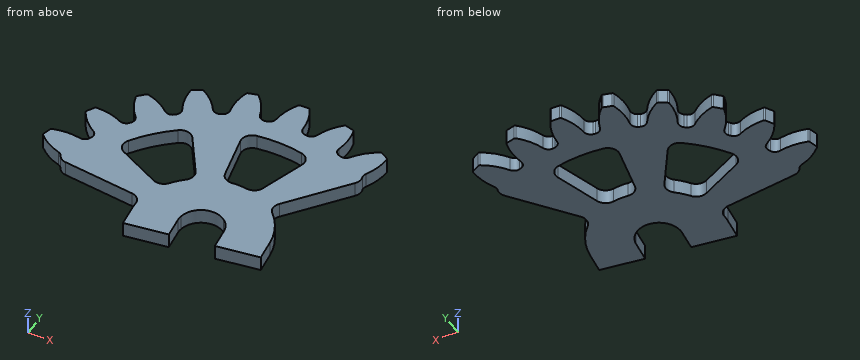
```python
from build123d import *

# Parameters (mm, degrees)
SKETCH3_R                = 136.611351841
EXTRUDE1_DEPTH           = 12.7
EXTRUDE2_DEPTH           = 12.7
FILLET2_R                = 1.5875
CIRPATTERN1_COUNT        = 24
FILLET2_OF_CIRPATTERN1_R = 1.5875
CUT_EXTRUDE1_DEPTH       = 234.890969431
CUT_EXTRUDE1_DEPTH_BACK  = 234.890969431
CUT_EXTRUDE2_REACH       = 232.646
SKETCH5_R                = 19.05
EXTRUDE3_DEPTH           = 12.7
CUT_EXTRUDE5_DEPTH       = 231.646456089
FILLET1_R                = 9.525
CUT_EXTRUDE7_DEPTH       = 12.7


with BuildPart() as part:
    # Sketch3 → Extrude1 (new body)
    with BuildSketch(Plane.XY):
        Circle(SKETCH3_R)
    extrude(amount=EXTRUDE1_DEPTH)

    # Sketch2 → Extrude2 (add)
    with BuildSketch(Plane.XY):
        with BuildLine():
            Line((-4.546074008, 165.141901983), (4.546074008, 165.141901983))
            ThreePointArc((4.546074008, 165.141901983), (9.719017906, 153.717756782), (11.846410355, 141.35876639))
            ThreePointArc((11.846410355, 141.35876639), (13.677789854, 137.226095775), (17.83135957, 135.442622788))
            Line((17.83135957, 135.442622788), (17.83135957, 110.042622788))
            Line((17.83135957, 110.042622788), (-17.83135957, 110.042622788))
            Line((-17.83135957, 110.042622788), (-17.83135957, 135.442622788))
            ThreePointArc((-17.83135957, 135.442622788), (-13.677789854, 137.226095775), (-11.846410355, 141.35876639))
            ThreePointArc((-11.846410355, 141.35876639), (-9.719017906, 153.717756782), (-4.546074008, 165.141901983))
        make_face()
    extrude2 = extrude(amount=EXTRUDE2_DEPTH)

    # Fillet2
    fillet2_edges = [part.edges().sort_by_distance(p)[0] for p in [
        (4.546074008, 165.141901983, 6.35),
        (-4.546074008, 165.141901983, 6.35),
    ]]
    fillet(fillet2_edges, radius=FILLET2_R)

    # CirPattern1: Extrude2 ×24 about axis
    cirpattern1_axis = Axis((0, 0, 0), (0, 0, 1))
    for i in range(1, CIRPATTERN1_COUNT):
        add(extrude2.rotate(cirpattern1_axis, i * 360 / CIRPATTERN1_COUNT))

    # Fillet2 of CirPattern1
    fillet2_of_cirpattern1_edges = [part.edges().sort_by_distance(p)[0] for p in [
        (-38.350699085, 160.691438662, 6.35),
        (-47.13303967, 158.338217595, 6.35),
        (-78.633935413, 145.290119351, 6.35),
        (-86.50796657, 140.744045343, 6.35),
        (-113.558398992, 119.987518509, 6.35),
        (-119.987518509, 113.558398992, 6.35),
        (-140.744045343, 86.50796657, 6.35),
        (-145.290119351, 78.633935413, 6.35),
        (-158.338217595, 47.13303967, 6.35),
        (-160.691438662, 38.350699085, 6.35),
        (-165.141901983, 4.546074008, 6.35),
        (-165.141901983, -4.546074008, 6.35),
        (-160.691438662, -38.350699085, 6.35),
        (-158.338217595, -47.13303967, 6.35),
        (-145.290119351, -78.633935413, 6.35),
        (-140.744045343, -86.50796657, 6.35),
        (-119.987518509, -113.558398992, 6.35),
        (-113.558398992, -119.987518509, 6.35),
        (-86.50796657, -140.744045343, 6.35),
        (-78.633935413, -145.290119351, 6.35),
        (-47.13303967, -158.338217595, 6.35),
        (-38.350699085, -160.691438662, 6.35),
        (-4.546074008, -165.141901983, 6.35),
        (4.546074008, -165.141901983, 6.35),
        (38.350699085, -160.691438662, 6.35),
        (47.13303967, -158.338217595, 6.35),
        (78.633935413, -145.290119351, 6.35),
        (86.50796657, -140.744045343, 6.35),
        (113.558398992, -119.987518509, 6.35),
        (119.987518509, -113.558398992, 6.35),
        (140.744045343, -86.50796657, 6.35),
        (145.290119351, -78.633935413, 6.35),
        (158.338217595, -47.13303967, 6.35),
        (160.691438662, -38.350699085, 6.35),
        (165.141901983, -4.546074008, 6.35),
        (165.141901983, 4.546074008, 6.35),
        (160.691438662, 38.350699085, 6.35),
        (158.338217595, 47.13303967, 6.35),
        (145.290119351, 78.633935413, 6.35),
        (140.744045343, 86.50796657, 6.35),
        (119.987518509, 113.558398992, 6.35),
        (113.558398992, 119.987518509, 6.35),
        (86.50796657, 140.744045343, 6.35),
        (78.633935413, 145.290119351, 6.35),
        (47.13303967, 158.338217595, 6.35),
        (38.350699085, 160.691438662, 6.35),
    ]]
    fillet(fillet2_of_cirpattern1_edges, radius=FILLET2_OF_CIRPATTERN1_R)

    # Sketch4 → Cut-Extrude1 (cut, two sides: drawn at the far end of the back side and taken through both)
    with BuildSketch(Plane.XY.offset(-CUT_EXTRUDE1_DEPTH_BACK)):
        Polygon((-1275.53694573, 167.92762467), (-268.218413087, 35.311623982), (0, 0), (164.689969961, 214.628147505), (783.198061827, 1020.683586133), (1560.818943381, -856.6592925), (-497.916064176, -1709.415253962), align=None)
    extrude(amount=CUT_EXTRUDE1_DEPTH + CUT_EXTRUDE1_DEPTH_BACK, mode=Mode.SUBTRACT)

    # Sketch5 → Cut-Extrude2 (cut, up to next)
    with BuildSketch(Plane.XY, mode=Mode.PRIVATE) as cut_extrude2_sk1:
        Circle(SKETCH5_R)
    cut_extrude2_tool1 = extrude(cut_extrude2_sk1.sketch, amount=CUT_EXTRUDE2_REACH, mode=Mode.PRIVATE) & part.part
    add(cut_extrude2_tool1.solids().sort_by_distance((0, 0, 0))[0], mode=Mode.SUBTRACT)

    # Sketch6 → Extrude3 (add)
    with BuildSketch(Plane.XY):
        with BuildLine():
            Line((-18.887024609, -2.486523962), (-16.400500647, -21.373548571))
            Line((-16.400500647, -21.373548571), (-54.174549866, -26.346596495))
            Line((-54.174549866, -26.346596495), (-56.661073828, -7.459571885))
            ThreePointArc((-56.661073828, -7.459571885), (-57.15, 0), (-56.661073828, 7.459571885))
            Line((-56.661073828, 7.459571885), (-18.887024609, 2.486523962))
            ThreePointArc((-18.887024609, 2.486523962), (-19.05, 0), (-18.887024609, -2.486523962))
        make_face()
        with BuildLine():
            Line((11.596905223, 15.113381133), (34.790715668, 45.340143398))
            ThreePointArc((34.790715668, 45.340143398), (49.493351826, 28.575), (56.661073828, 7.459571885))
            Line((56.661073828, 7.459571885), (59.147597789, -11.427452724))
            Line((59.147597789, -11.427452724), (21.373548571, -16.400500647))
            Line((21.373548571, -16.400500647), (18.887024609, 2.486523962))
            ThreePointArc((18.887024609, 2.486523962), (16.497783942, 9.525), (11.596905223, 15.113381133))
        make_face()
    extrude(amount=EXTRUDE3_DEPTH)

    # Sketch8 → Cut-Extrude5 (cut, through all)
    with BuildSketch(Plane.XY):
        with BuildLine():
            Line((-25.426243647, 114.690373436), (-12.369523937, 55.795316807))
            ThreePointArc((-12.369523937, 55.795316807), (2.492847988, 57.095605863), (17.185336442, 54.504923735))
            Line((17.185336442, 54.504923735), (35.325413797, 112.037898789))
            ThreePointArc((35.325413797, 112.037898789), (5.124187531, 117.36318983), (-25.426243647, 114.690373436))
        make_face()
        with BuildLine():
            Line((-63.119271491, 99.077410097), (-30.706672617, 48.199821128))
            ThreePointArc((-30.706672617, 48.199821128), (-42.135399799, 38.609980365), (-50.692669116, 26.388933246))
            Line((-50.692669116, 26.388933246), (-104.201597628, 54.24391834))
            ThreePointArc((-104.201597628, 54.24391834), (-86.611655142, 79.36495964), (-63.119271491, 99.077410097))
        make_face()
    extrude(amount=CUT_EXTRUDE5_DEPTH, mode=Mode.SUBTRACT)

    # Fillet1
    fillet1_edges = [part.edges().sort_by_distance(p)[0] for p in [
        (34.790715668, 45.340143398, 6.35),
        (-50.692669116, 26.388933246, 6.35),
        (-30.706672617, 48.199821128, 6.35),
        (-63.119271491, 99.077410097, 6.35),
        (-104.201597628, 54.24391834, 6.35),
        (-12.369523937, 55.795316807, 6.35),
        (17.185336442, 54.504923735, 6.35),
        (35.325413797, 112.037898789, 6.35),
        (-25.426243647, 114.690373436, 6.35),
        (-56.661073828, 7.459571885, 6.35),
    ]]
    fillet(fillet1_edges, radius=FILLET1_R)

    # Sketch9 → Cut-Extrude7 (cut)
    with BuildSketch(Plane.XY):
        with BuildLine():
            Line((79.034097122, 102.999240689), (83.809524096, 109.222698287))
            Line((83.809524096, 109.222698287), (80.539107883, 111.732176909))
            ThreePointArc((80.539107883, 111.732176909), (80.864034333, 107.180027092), (79.034097122, 102.999240689))
        make_face()
        with BuildLine():
            Line((-128.717007568, 16.945915528), (-136.494393434, 17.969827802))
            Line((-136.494393434, 17.969827802), (-135.956329304, 22.056830634))
            ThreePointArc((-135.956329304, 22.056830634), (-132.967230996, 18.608216933), (-128.717007568, 16.945915528))
        make_face()
    extrude(amount=CUT_EXTRUDE7_DEPTH, mode=Mode.SUBTRACT)


solid = part.part
```
Input: part model. Units: mm. Frame: model coordinates. Coordinates: 2 decimals unless noted, no trailing zeros. Loops run counter-clockwise (first coordinate to the right, second up) from the corner with the lowest first, then second, coordinate; pieces in that order, holes last. Notation, with made-up numbers: M 80.5,17.25 L 92.5,17.25 A17 cw 92.5,49.25 Z; hole C 3,31.25 d10. An arc over 180 degrees is marked long. Answer in a Markdown table with one row per item.
1. First-contact query: pin 1 (5 mm diameter, centred on x = -116, z = 6, fed in from -Y); pin 2 (12 mm diameter, centred on x = 2.5, y = 65.5, fed in from -Z); pin 3 (4 mm diameter, centred on x = 20, z = 11, fed in from +Y); pin 4 (3 mm diameter, centred on y = 11.5, z = 3.5, fed in from +X). Flat tips, straight axial feed; report the tip coordinate or a pass-through.
Response:
| item | result |
|---|---|
| pin 1 | stops at y = 14.94 |
| pin 2 | passes through |
| pin 3 | stops at y = 135.93 |
| pin 4 | stops at x = 56.27 |
2. Section A-A, the plane y = 148. Output: boundary loops of the cut face in (x, z).
Response:
| item | result |
|---|---|
| outline | M -49.06,0 L -28.66,0 L -28.66,12.7 L -49.06,12.7 Z; M -11.11,0 L 11.11,0 L 11.11,12.7 L -11.11,12.7 Z; M 28.66,0 L 49.06,0 L 49.06,12.7 L 28.66,12.7 Z |
3. Section B-B, the plane y = 71. Output: boundary loops of the cut face in (x, z), then the cut area to 3 significant figures.
Response:
| item | result |
|---|---|
| outline | M -140.2,0 L -93.59,0 L -93.59,12.7 L -140.2,12.7 Z; M -45.23,0 L -15.74,0 L -15.74,12.7 L -45.23,12.7 Z; M 22.39,0 L 54.48,0 L 54.48,12.7 L 22.39,12.7 Z |
| area | 1,370 mm2 |
4. Section D-D, the plane x = 64. Output: boundary loops of the cut face in (y, z), then the cut area to 3 significant figures.
Response:
| item | result |
|---|---|
| outline | M 83.41,0 L 133.27,0 L 133.27,12.7 L 83.41,12.7 Z |
| area | 633 mm2 |
5. Material intervals for line 1 (X direction, y = 151, z = 12.25); line 2 (X direction, y = 141.5, z = 8.5); line 3 (X direction, y = 91.5, z = 1.25), sorted ascending.
Response:
| item | result |
|---|---|
| line 1 | x = -48.73 to -30.4, -10.47 to 10.47, 30.4 to 48.73 |
| line 2 | x = -85.2 to -72.67, -49.13 to -25.78, -11.84 to 11.84, 25.78 to 49.13, 72.67 to 85.2 |
| line 3 | x = -108.26 to -73.68, -58.35 to -20.29, 28.85 to 70.21 |
6. Section C-C, the plane z = 10.75. Count the separate pieces of the cut face and the enclosed holes in it, then the cut area to 3 significant figures.
Response:
| item | result |
|---|---|
| separate pieces | 1 |
| enclosed holes | 2 |
| area | 21,400 mm2 |
